Geometry: see drawing. Coordinates: mm, zero at the bounding-box minimum. Coordinates: 2 decimals unless noted, no trailing zeros. Loops run counter-clockwise (first coordinate to the right, second up) from the corner with the lowest first, then second, coordinate; pieces in that order, holes last. Notation, with made-up numbers: M 43,43.25 L 101,43.25 A31 ccw 101,79.25 Z; hole C 25,13.5 d6. An arc over 180 degrees is marked long. One line per question, with ' | ' between items. Start each with the question number.
1. Pin query (flat end, axial travel): P1, Ø3, axis at x = 6, y = 2, coming from the -Z side; P2, Ø2.5, axis at x = 12.7, z = 7.62, coming from the +Y side; P3, Ø1.5, axis at x = 15.5, y = 4.5, coming from the -Z side; P4, Ø3, axis at x = 8, y = 5.5, coming from the +Z side. Return the tip coordinate at first contact, or that it passes through.
2. Section query C-C, the plane x = 10. Output: boundary loops of the cut face in (y, z).
3. Section query D-D, the plane y = 1.25. Output: boundary loops of the cut face in (x, z) (1 decimal).
4. Ray query, probe 1 along Z at (x, y) = (12.7, 1.5) (1 decimal); probe 2 along Z at (x, y) = (11.75, 4) (1 decimal); probe 3 along X at (y, z) = (5.75, 11) (1 decimal). Return the intervals inside material, ascending.
5. Section query B-B, the plane x = 12.7. State how many separate pieces and enclosed holes the cut face has, and give its area (3 significant figures).
6. Section query A-A, the plane z = 12.7. Output: boundary loops of the cut face in (x, y), and give its area (3 significant figures).
7. Mould query, pull axis Z, two halves, no side actions, for the marked faces 1, 2, 3 and 4. Classes: pulls with the +Z half, pulls with the -Z half, needs draft (parallel to the pull), parting line crosses it, or undercut.
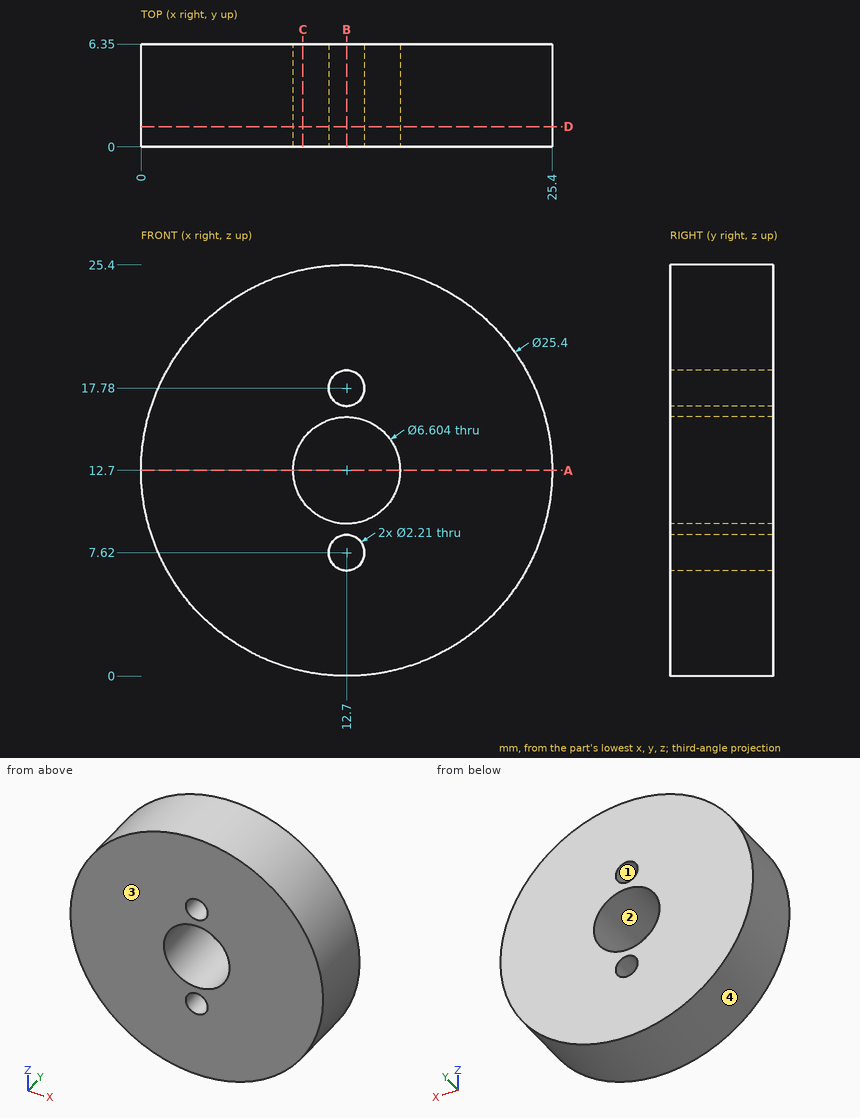
Taken from the geometry:
1) P1: z = 1.11 | P2: y = 6.35 | P3: z = 0.17 | P4: z = 24.99
2) outline: M 0,0.29 L 6.35,0.29 L 6.35,10.8 L 0,10.8 Z; M 0,14.6 L 6.35,14.6 L 6.35,25.11 L 0,25.11 Z
3) outline: C 12.7,12.7 d25.4; hole C 12.7,12.7 d6.6; hole C 12.7,7.6 d2.2; hole C 12.7,17.8 d2.2
4) probe 1: 0 to 6.5, 8.7 to 9.4, 16 to 16.7, 18.9 to 25.4 | probe 2: 0 to 7.1, 8.2 to 9.5, 15.9 to 17.2, 18.3 to 25.4 | probe 3: 0.1 to 9.9, 15.5 to 25.3
5) separate pieces: 4 | enclosed holes: 0 | area: 91.3 mm^2
6) outline: M 0,0 L 9.4,0 L 9.4,6.35 L 0,6.35 Z; M 16,0 L 25.4,0 L 25.4,6.35 L 16,6.35 Z | area: 119 mm^2
7) face 1: undercut | face 2: undercut | face 3: needs draft | face 4: parting line crosses it
